from build123d import *

# Parameters (mm, degrees)
SKIZZE1_W                       = 7.5
SKIZZE1_H                       = 5
AUFSATZ_LINEAR_AUSTRAGEN1_DEPTH = 5
AUFSATZ_LINEAR_AUSTRAGEN2_DEPTH = 5


with BuildPart() as part:
    # Skizze1 → Aufsatz-Linear austragen1 (new body)
    with BuildSketch(Plane.XY):
        Rectangle(SKIZZE1_W, SKIZZE1_H)
    extrude(amount=AUFSATZ_LINEAR_AUSTRAGEN1_DEPTH)

    # Skizze2 → Aufsatz-Linear austragen2 (add)
    with BuildSketch(Plane(origin=(0, 0, 0), x_dir=(-1, 0, 0), z_dir=(0, 0, -1))):
        with BuildLine():
            ThreePointArc((-0.375, 0), (-1.875, 1.5), (-3.375, 0))
            Line((-3.375, 0), (-0.375, 0))
        make_face()
        with BuildLine():
            Line((-0.375, 0), (-3.375, 0))
            ThreePointArc((-3.375, 0), (-1.875, -1.5), (-0.375, 0))
        make_face()
    extrude(amount=AUFSATZ_LINEAR_AUSTRAGEN2_DEPTH)


solid = part.part
Geometry check sheet. Reference: the model listing, model coordinates, mm. A direction names the side the tool comes from. Round coordinates to 2 decimals unless told otherwise and drop trailing zeros. Order: outer loops, then holes, each group sorted by start corner. A loop starts at its lowest first (then second) coordinate and runs counter-clockwise, first axis right, second up. Notation, with made-up numbers: M 51.25,-13 L 82.25,-13 A17 cw 82.25,16 Z; hole C 9.25,-6.75 d1. An arc over 180 degrees is marked long. Answer in a Markdown table with one row per item.
(1) Sectioned sample at B-B, the plane z = -2. Record the cut outline in (x, y) (3 decimals), and give its area (3 significant figures).
Responses:
| item | result |
|---|---|
| outline | C 1.875,0 d3 |
| area | 7.07 mm² |
(2) Go/stop test with a flat-tipped pin: P1, Ø1.5, axis at x = 1.5, z = -1.5, coming from the -Y side. Record where the tip stops, or that it passes through.
Responses:
| item | result |
|---|---|
| P1 | stops at y = -1.5 |
(3) Sectioned sample at D-D, the plane y = 1.8. Record the cut outline in (x, z).
Responses:
| item | result |
|---|---|
| outline | M -3.75,0 L 3.75,0 L 3.75,5 L -3.75,5 Z |
(4) Tool access check on faces 1 (the face through (0.376, -0.066, -2.465)), 2 (the face through (0, 2.5, 2)). Record the directions out of +Z, -Z, +X, -X, +Y, -Y that give a thin tool (end or side, any length) a straight path to the whole face; none if there is none.
Responses:
| item | result |
|---|---|
| face 1 | -Z |
| face 2 | +Z, -Z, +X, -X, +Y |
(5) Sectioned sample at A-A, the plane y = 0. Record the cut outline in (x, z) (3 decimals).
Responses:
| item | result |
|---|---|
| outline | M -3.75,0 L 0.375,0 L 0.375,-5 L 3.375,-5 L 3.375,0 L 3.75,0 L 3.75,5 L -3.75,5 Z |
(6) Scan lines: probe 1 along Z at (x, y) = (-1.5, 1.65); probe 2 along Y at (x, z) = (1.5, -2.25); probe 3 along Y at (x, z) = (1.25, -4.5). Record each from-to range of solid material in increasing order. Write a range as from..to.
Responses:
| item | result |
|---|---|
| probe 1 | z = 0..5 |
| probe 2 | y = -1.45..1.45 |
| probe 3 | y = -1.36..1.36 |
(7) Sectioned sample at C-C, the plane x = 0.5. Record the cut outline in (y, z), and give its area (3 significant figures).
Responses:
| item | result |
|---|---|
| outline | M -2.5,0 L -0.6,0 L -0.6,-5 L 0.6,-5 L 0.6,0 L 2.5,0 L 2.5,5 L -2.5,5 Z |
| area | 31.0 mm² |
